Design review of the part shown in the three views and the two pictorial views. Dimensions are in mm from the part's minimum x, y and z. Give positions to 0.01 mm unless a question says otherwise; leave off trailing zeros. Loops run counter-clockwise (first coordinate to the right, second up) from the corner with the lowest first, then second, coordinate; pieces in that order, holes last. Notation, with made-up numbers: (17.25, 29.5) -> (26.25, 29.5) arc R29 ccw to (26.25, 68.5) -> close; hole circle Ø3 at (70, 5). An arc over 180 degrees is marked (long way). Use CSV: the item, a comma, the result in double quotes. Start each with the question number.
Item 1: We need section A-A (x = 26). State the section outline as (y, z) points, plus the area to 3 significant figures.
Item 2: We need section C-C (y = 23). State the section outline as (x, z) points, plus the area to 3 significant figures.
Item 3: Clearance check with flat-ended pins moving along their axes: pin 1 (3 mm diameter, centred on x = 25, z = 1.5, fed in from +Y); pin 2 (12 mm diameter, centred on x = 24.5, y = 24.5, fed in from +Z); pin 3 (1 mm diameter, centred on x = 6, z = 6, fed in from +Y). State where each tip first meets the part, or that it passes through.
Item 4: We need section D-D (x = 51). State the section outline as (y, z) points, plus the area to 3 significant figures.
Item 5: We need section B-B (z = 1.75). State the section outline as (x, y) points.
Item 6: The part is to be moulded in two halves that separate along Y. For the marked faces 1, 2 and 3, say which applies: +Y half, -Y half, draft (parallel to the pull), parting line (faces both ways), or undercut.
Item 7: Wall thickness on line 1 along Y through (x, z) = (28, 4.5); line 2 along X through (y, z) = (65.5, 3.25); line 3 along Y through (x, z) = (37.5, 2): over which ranges is each line inside the solid? List them lowest first. Write a range as from..to.
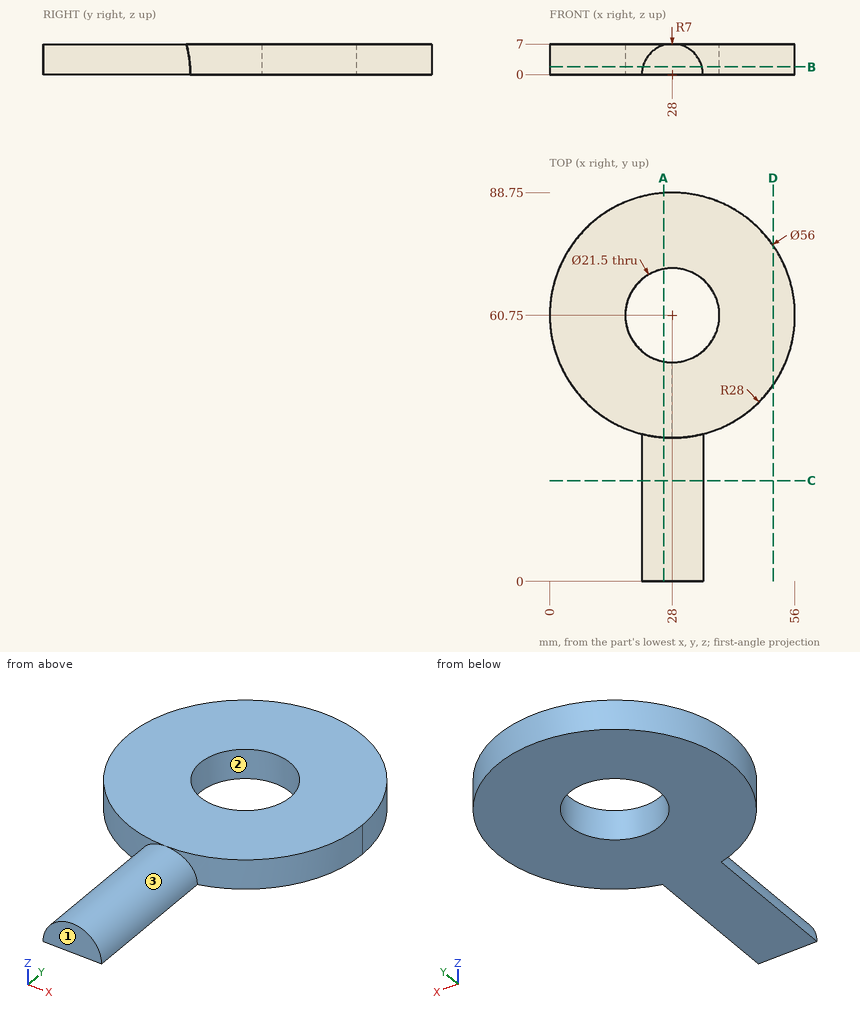
Results found:
1,outline,"(0, 0) -> (50.19, 0) -> (50.19, 7) -> (32.82, 7) -> (32.82, 6.71) -> (0, 6.71) -> close; (71.31, 0) -> (88.68, 0) -> (88.68, 7) -> (71.31, 7) -> close"
1,area,"463 mm²"
2,outline,"(21, 0) -> (35, 0) arc R7 ccw to start"
2,area,"77.0 mm²"
3,pin 1,"y = 88.71"
3,pin 2,"z = 7"
3,pin 3,"y = 78.69"
4,outline,"(44.78, 0) -> (76.72, 0) -> (76.72, 7) -> (44.78, 7) -> close"
4,area,"224 mm²"
5,outline,"(21.22, 0) -> (34.78, 0) -> (34.78, 33.58) arc R28 ccw (long way) to (21.22, 33.58) -> close; hole circle Ø21.5 at (28, 60.75)"
6,face 1,"-Y half"
6,face 2,"undercut"
6,face 3,"draft"
7,line 1,"0..50, 71.5..88.75"
7,line 2,"0.41..18.36, 37.64..55.59"
7,line 3,"34.41..55.72, 65.78..87.09"
